Geometry: final body of the model. Coordinates: model frame, mm. Give positions to 0.01 mm unless a question says otherwise; leave off trailing zeros. Order: outer loops, then holes, each group sorted by start corner. A loop starts at its lowest first (then second) coordinate and runs counter-clockwise, first axis right, second up. Notation, with made-up numbers: M 21,-27.75 L 36,-27.75 A25 ccw 36,-0.75 Z; hole C -13,55.25 d9. An arc over 180 degrees is marked long. Use CSV: the item, a comma, the result in double quotes.
```python
from build123d import *

# Parameters (mm, degrees)
F0_R     = 2.15265
F1_DEPTH = 3.175


with BuildPart() as f1:
    # F0 (on Top) → F1 (new body)
    with BuildSketch(Plane.XY):
        with BuildLine():
            ThreePointArc((393.7, 0), (196.85, 196.85), (0, 0))
            Line((0, 0), (0, -139.7))
            ThreePointArc((0, -139.7), (196.85, -336.55), (393.7, -139.7))
            Line((393.7, -139.7), (393.7, 0))
        make_face()
        with Locations((133.547731, -176.317746)):
            Circle(F0_R, mode=Mode.SUBTRACT)
        with Locations((269.08125, -254)):
            Circle(F0_R, mode=Mode.SUBTRACT)
        with Locations((327.81875, -254)):
            Circle(F0_R, mode=Mode.SUBTRACT)
        with Locations((269.08125, -195.2625)):
            Circle(F0_R, mode=Mode.SUBTRACT)
        with Locations((260.152269, -176.317746)):
            Circle(F0_R, mode=Mode.SUBTRACT)
        with Locations((327.81875, -195.2625)):
            Circle(F0_R, mode=Mode.SUBTRACT)
        with Locations((133.547731, 62.017746)):
            Circle(F0_R, mode=Mode.SUBTRACT)
        with Locations((260.152269, 62.017746)):
            Circle(F0_R, mode=Mode.SUBTRACT)
        with Locations((196.85, 96.8375)):
            Circle(F0_R, mode=Mode.SUBTRACT)
        with Locations((196.85, 173.0375)):
            Circle(F0_R, mode=Mode.SUBTRACT)
    extrude(amount=F1_DEPTH)


solid = f1.part
```
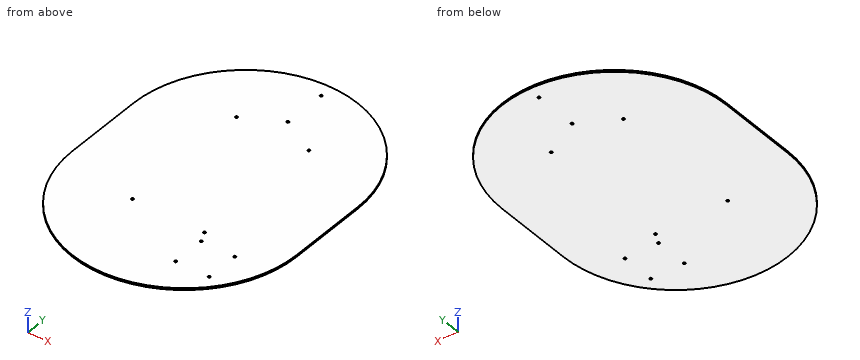
1. Line query: line 1 (Y direction, x = 196.85, z = 2.5); line 2 (X direction, y = -177, z = 2.1); line 3 (Y direction, x = 198, z = 1.25). Output: solid intervals per line, ascending.
Answer:
line 1,"-336.55 to 94.68, 98.99 to 170.88, 175.19 to 196.85"
line 2,"3.57 to 131.51, 135.59 to 258.11, 262.19 to 390.13"
line 3,"-336.55 to 95.02, 98.66 to 171.22, 174.86 to 196.85"
2. Section A-A, the plane z = 2.2. Give the number of separate pieces and of enclosed holes in the cut face, plus the area to 3 significant figures.
Answer:
separate pieces,"1"
enclosed holes,"10"
area,"177,000 mm2"
3. Section B-B, the plane y = -269. Return the cut outline in (x, z) (3 decimals).
Answer:
outline,"M 48.42,0 L 345.28,0 L 345.28,3.175 L 48.42,3.175 Z"
4. Section C-C, the plane x = 51. Return the cut outline in (y, z) (3 decimals).
Answer:
outline,"M -271.903,0 L 132.203,0 L 132.203,3.175 L -271.903,3.175 Z"
